from build123d import *

# Parameters (mm, degrees)
SKETCH1_W           = 245.11
SKETCH1_H           = 15.24
BOSS_EXTRUDE1_DEPTH = 3.175
FILLET2_R           = 7.62
SKETCH3_R           = 1.4605
CUT_EXTRUDE1_DEPTH  = 123.832703504


with BuildPart() as part:
    # Sketch1 → Boss-Extrude1 (new body)
    with BuildSketch(Plane.XY):
        Rectangle(SKETCH1_W, SKETCH1_H)
    extrude(amount=BOSS_EXTRUDE1_DEPTH)

    # Fillet2
    fillet2_edges = [part.edges().sort_by_distance(p)[0] for p in [
        (-122.555, -7.62, 1.5875),
        (-122.555, 7.62, 1.5875),
        (122.555, -7.62, 1.5875),
        (122.555, 7.62, 1.5875),
    ]]
    fillet(fillet2_edges, radius=FILLET2_R - 0.0001)  # a hair under: the kernel refuses the full size

    # Sketch3 → Cut-Extrude1 (cut, through all)
    with BuildSketch(Plane.XY.offset(3.175)):
        with Locations((-114.935, 0)):
            Circle(SKETCH3_R)
        with Locations((114.935, 0)):
            Circle(SKETCH3_R)
        Circle(SKETCH3_R)
    extrude(amount=-CUT_EXTRUDE1_DEPTH, mode=Mode.SUBTRACT)


solid = part.part
Could you check a few things on this model? Use its own coordinates, in mm. Give positions to 0.01 mm unless a question says otherwise; leave off trailing zeros. Loops run counter-clockwise (first coordinate to the right, second up) from the corner with the lowest first, then second, coordinate; pieces in that order, holes last. Notation, with made-up numbers: M 22.5,39.5 L 54.5,39.5 A10 cw 54.5,53.5 Z; hole C -10.5,39.5 d2. An arc over 180 degrees is marked long. Answer as a JSON object with one key per item and string values.
Q1. If I drill on probe 1 along X at (y, z) = (1.25, 2.25); probe 2 along Y at (x, z) = (0, 2.2); probe 3 along X at (y, z) = (1.5, 0.4), over which ranges is the centre line in solid material (lowest first)? Write a range as [from, to].
Values found:
{"probe 1": "x = [-122.45, -115.69], [-114.18, -0.76], [0.76, 114.18], [115.69, 122.45]", "probe 2": "y = [-7.62, -1.46], [1.46, 7.62]", "probe 3": "x = [-122.41, 122.41]"}
Q2. Suppose I cut it at A-A, the plane z = 2.2. State how many separate pieces and enclosed holes the cut face has, plus the area to 3 significant figures.
Values found:
{"separate pieces": "1", "enclosed holes": "3", "area": "3,670 mm²"}
Q3. For P1, Ø2.5, axis at x = -114.935, y = 0, coming from the +Z side, with a flat end and sliding along its axis, tell me the tip position at first contact or that it passes through.
Values found:
{"P1": "passes through"}
Q4. Suppose I cut it at B-B, the plane y = 5.5. List the corners of the cut face in (x, z) for me (3 decimals).
Values found:
{"outline": "M -120.209,0 L 120.209,0 L 120.209,3.175 L -120.209,3.175 Z"}
